Autodesk Inventor part; units mm, degrees
ref_plane "YZ Plane" through (0, 0, 0) normal (1, 0, 0) x (0, 1, 0)
ref_plane "XZ Plane" through (0, 0, 0) normal (0, 1, 0) x (-1, 0, 0)
ref_plane "XY Plane" through (0, 0, 0) normal (0, 0, 1) x (1, 0, 0)
sketch "Sketch1" plane through (0, 0, 0) normal (0, 0, 1) x (1, 0, 0)
  point P0 (0, 0)
sketch "Sketch2" plane through (0, 0, 0) normal (0, 0, 1) x (1, 0, 0)
  line L0 (-27.5, 7.5) -> (27.5, 7.5)
  line L1 (27.5, 7.5) -> (27.5, -7.5)
  line L2 (27.5, -7.5) -> (-27.5, -7.5)
  line L3 (-27.5, -7.5) -> (-27.5, 7.5)
  line L4 (-27.5, 7.5) -> (27.5, -7.5) construction
  line L5 (27.5, 7.5) -> (-27.5, -7.5) construction
  point P0 (0, 0)
  dimension "d0" = 15
  dimension "d1" = 55
extrude "Extrusion1" add sketch "Sketch2" along normal blind 3
sketch "Sketch3" plane through (0, 0, 3) normal (0, 0, 1) x (1, 0, 0)
  line L0 (0, 0) -> (22.5765, 0) construction
  circle A0 centre (22.5765, 0) radius 1.75
  line L1 (27.5, 7.5) -> (-27.5, 7.5) construction
  line L2 (0, 7.5) -> (0, -7.5) construction
  line L3 (-27.5, -7.5) -> (27.5, -7.5) construction
  line L4 (0, 0) -> (-22.5765, 0) construction
  circle A1 centre (-22.5765, 0) radius 1.75
  dimension "d4" = 3.5
  dimension "d5" = 45.153
extrude "Extrusion2" cut sketch "Sketch3" against normal through all
sketch "Sketch4" plane through (-27.5, 7.5, 0) normal (0, 1, 0) x (1, 0, 0)
  line L0 (55, 0) -> (0, 0)
  line L1 (19, 0) -> (19, 10.8562)
  line L2 (36, 0) -> (36, 10.8562)
  line L3 (27.5, 10.8562) -> (27.5, 0) construction
  line L4 (19, 7.8562) -> (36, 7.8562) construction
  line L5 (19, 0) -> (36, 0) construction
  line L6 (19, 0) -> (36, 0)
  line L7 (19, 10.8562) -> (36, 10.8562) construction
  circle A0 centre (27.5, 13.8562) radius 6
  line L8 (19, 10.8562) -> (22.3038, 10.8562)
  line L9 (36, 10.8562) -> (32.6962, 10.8562)
  dimension "d10" = 10.8562
  dimension "d11" = 17
  dimension "d12" = 12
  dimension "d13" = 3
extrude "Extrusion3" add sketch "Sketch4" against normal up to surface (15 mm away) contours L0 L1 L8 A0 L9 L2
fillet "Fillet1" radius 3 4 edges at (-27.5, 7.5, 1.5) (-27.5, -7.5, 1.5) (27.5, 7.5, 1.5) (27.5, -7.5, 1.5)
fillet "Fillet2" radius 2 8 edges at (-26.6213, 6.6213, 3) (-27.5, 0, 3) (-26.6213, -6.6213, 3) (0, -7.5, 3) (26.6213, -6.6213, 3) (27.5, 0, 3) (26.6213, 6.6213, 3) (0, 7.5, 3)
fillet "Fillet3" radius 5 2 edges at (-8.5, 0, 0) (8.5, 0, 0)
fillet "Fillet4" radius 2 6 edges at (-6.8481, 7.5, -10.8562) (-8.5, 0, -10.8562) (8.5, 0, -10.8562) (-6.8481, -7.5, -10.8562) (6.8481, -7.5, -10.8562) (6.8481, 7.5, -10.8562)
properties part number "PlotterPenHolderAltClamp"
The model under review builds one solid part; all positions refer to its coordinate system, in mm. A direction names the side the tool comes from. Round coordinates to 2 decimals unless told otherwise and drop trailing zeros. Loops run counter-clockwise (first coordinate to the right, second up) from the corner with the lowest first, then second, coordinate; pieces in that order, holes last. Notation, with made-up numbers: M 11.5,-37 L 58.5,-37 A13 ccw 58.5,-12 Z; hole C 34,37.25 d7. An arc over 180 degrees is marked long. Answer as CSV lines item,"result". Start each with the question number.
Item 1: Consider section D-D (x = -7). Write out the cut boundary in (y, z), then the cut area to 3 significant figures.
Item 2: Consider section A-A (x = 22). Write out the cut boundary in (y, z).
Item 3: Insertion check: P1, Ø1.5, axis at y = -4.5, z = -7, coming from the +X side; P2, Ø1, axis at y = 3.5, z = -4, coming from the -X side; P3, Ø1, axis at x = 12, z = -1.5, coming from the -Y side; P4, Ø2, axis at y = 4.5, z = -7, coming from the -X side. Each pin has a flat end and moves straight along its axis. Give the tip position at first contact, or say it passes through.
Item 4: For faces 1 (the face through (-0.088, 0.105, -7.857)), 2 (the face through (-8.5, 0, -7)), list the 3-axis set-ups (+Z, -Z, +X, -X, +Y, -Y) from which the entire face can be reached by the end or side of a thin tool; tool diameter is ignored.
Item 5: Wall thickness on line 1 (Z direction, x = -21.5, y = 1.5); line 2 (X direction, y = -7, z = -8.75); line 3 (X direction, y = -5.5, z = -9.75): over which ranges is each line inside the solid? List them lowest first. Write a range as [from, to].
Item 6: Consider section B-B (y = 0). Write out the cut boundary in (x, z), then the cut area to 3 significant figures.
Item 7: Consider section C-C (y = -3.25). Write out the cut boundary in (x, z).
Item 8: Mouldability with a two-part tool opening along X and no side actions: class faces 3 (the face through (-9.93, -0.11, -1.5)), 4 (the face through (24.246, 0.526, 1.521)), 5 (the face through (-6, 0, -10.856)) as released by +X, released by -X, zero draft, split by the parting line, or undercut.
Answer:
1,outline,"M -7.5,-8.86 A2 ccw -6,-10.79 L 6,-10.79 A2 ccw 7.5,-8.86 L 7.5,1 A2 ccw 5.5,3 L -5.5,3 A2 ccw -7.5,1 Z"
1,area,"204 mm^2"
2,outline,"M -7.5,0 L -1.65,0 L -1.65,3 L -5.5,3 A2 ccw -7.5,1 Z; M 1.65,0 L 7.5,0 L 7.5,1 A2 ccw 5.5,3 L 1.65,3 Z"
3,P1,"stops at x = 8.5"
3,P2,"stops at x = -8.73"
3,P3,"passes through"
3,P4,"stops at x = -8.5"
4,face 1,"-Z, +Y, -Y"
4,face 2,"-Z, -X, +Y, -Y"
5,line 1,"z = [0, 3]"
5,line 2,"x = [-8.5, -3.15], [3.15, 8.5]"
5,line 3,"x = [-8.29, -4.37], [4.37, 8.29]"
6,outline,"M -27.5,0 L -24.33,0 L -24.33,3 L -25.5,3 A2 ccw -27.5,1 Z; M -20.83,0 L -13.5,0 A5 cw -8.5,-5 L -8.5,-8.86 A2 ccw -6.5,-10.86 L -5.2,-10.86 A6 cw 5.2,-10.86 L 6.5,-10.86 A2 ccw 8.5,-8.86 L 8.5,-5 A5 cw 13.5,0 L 20.83,0 L 20.83,3 L -20.83,3 Z; M 24.33,0 L 27.5,0 L 27.5,1 A2 ccw 25.5,3 L 24.33,3 Z"
6,area,"314 mm^2"
7,outline,"M -27.5,0 L -13.5,0 A5 cw -8.5,-5 L -8.5,-8.86 A2 ccw -6.5,-10.86 L -5.2,-10.86 A6 cw 5.2,-10.86 L 6.5,-10.86 A2 ccw 8.5,-8.86 L 8.5,-5 A5 cw 13.5,0 L 27.5,0 L 27.5,1 A2 ccw 25.5,3 L -25.5,3 A2 ccw -27.5,1 Z"
8,face 3,"released by -X"
8,face 4,"undercut"
8,face 5,"zero draft"
